Input: part model. Units: mm. Frame: model coordinates. A direction names the side the tool comes from. Give positions to 0.01 mm unless a question says otherwise; leave off trailing zeros. Loops run counter-clockwise (first coordinate to the right, second up) from the corner with the lowest first, then second, coordinate; pieces in that order, holes last. Notation, with made-up numbers: (65, 49) - (84, 49) arc R22 ccw to (84, 76) - close; hole circle Ø10 at (82.25, 60). An arc over 180 degrees is marked (long way). Answer as a JSON object with one key per item and string values.
from build123d import *

# Parameters (mm, degrees)
F1_DEPTH = 288
F3_DEPTH = 304
F5_W     = 50.8
F5_H     = 304
F6_DEPTH = 36
F7_W     = 75.9582033121
F7_H     = 107.4988492727
F8_DEPTH = 100
F9_R     = 10


with BuildPart() as f1:
    # F0 (on Front) → F1 (new body)
    with BuildSketch(Plane.XZ):
        Polygon((0, 48.8444454968), (0, 0), (134.5802352905, 0), (134.5802352905, 40), (62.8, 64.8444454968), (50.8, 64.8444454968), (50.8, 48.8444454968), align=None)
    extrude(amount=F1_DEPTH)

    # F2 (on Front) → F3 (join)
    with BuildSketch(Plane.XZ):
        Polygon((0, 0), (134.5802352905, 0), (134.5802352905, 40), (62.8, 64.8444454968), (0, 64.8444454968), align=None)
    extrude(amount=-F3_DEPTH)

    # F5 (on face) → F6 (join)
    with BuildSketch(Plane.XY.offset(64.8444454968)):
        with Locations((25.4, 152)):
            Rectangle(F5_W, F5_H)
    extrude(amount=F6_DEPTH)

    # F7 (on face) → F8 (join)
    with BuildSketch(Plane(origin=(26.7612103496, 0, 77.3181263313), x_dir=(0.944996487, 0, -0.3270804787), z_dir=(0.3270804787, 0, 0.944996487))):
        with Locations((76.1155287701, 250.2505753636)):
            Rectangle(F7_W, F7_H)
    extrude(amount=F8_DEPTH)

    # F9
    f9_edges = [f1.edges().sort_by_distance(p)[0] for p in [
        (62.8, 250.250575, 64.844445),
    ]]
    fillet(f9_edges, radius=F9_R)


solid = f1.part
Item 1: Cut plane C-C (z = 83). Return loops of the section in (x, y).
Geometry check:
{"outline": "(0, 0) - (50.8, 0) - (50.8, 304) - (0, 304) - close; (69.08, 196.5) - (149.46, 196.5) - (149.46, 304) - (69.08, 304) - close"}
Item 2: Access query for faces 5 (the face through (119, 196.501, 96)), 6 (the face through (25, 154, 100.844)), 7 (the face through (50.8, -142, 57)), 8 (the face through (134.58, 4, 20)). Directions: +Z, -Z, +X, -X, +Y, -Y. A direction counts if a zero-diameter tool reaches every point of the face in a straight line with its end or side. Return the directions, or none.
Geometry check:
{"face 5": "+Z, +X, -Y", "face 6": "+Z, -X, +Y, -Y", "face 7": "+Z, -X, -Y", "face 8": "-Z, +X, +Y, -Y"}
Item 3: Cut plane B-B (x = 11). Return loops of the section in (y, z).
Geometry check:
{"outline": "(-288, 0) - (304, 0) - (304, 100.84) - (0, 100.84) - (0, 48.84) - (-288, 48.84) - close"}
Item 4: Cut plane A-A (y = -249). Return loops of the section in (x, z), then the cut area to 3 significant figures.
Geometry check:
{"outline": "(0, 0) - (134.58, 0) - (134.58, 40) - (62.8, 64.84) - (50.8, 64.84) - (50.8, 48.84) - (0, 48.84) - close", "area": "7,020 mm2"}
Item 5: Cut plane D-D (z = 30.5). Return loops of the section in (x, y), then the cut area to 3 significant figures.
Geometry check:
{"outline": "(0, -288) - (134.58, -288) - (134.58, 304) - (0, 304) - close", "area": "79,700 mm2"}
Item 6: Contact query for flat-ended pins moving along their axis: P1, Ø8, axis at x = 69, y = 29, coming from the +Z side; P2, Ø9.5, axis at x = 55.5, y = -29.5, coming from the +Z side; P3, Ø6, axis at x = 89.5, y = -53, coming from the +Z side. Output: stop coordinate, or through.
Geometry check:
{"P1": "stops at z = 64.08", "P2": "stops at z = 64.84", "P3": "stops at z = 56.64"}
Item 7: Material intervals for line 1 (Z direction, x = 31, y = -235); line 2 (X direction, y = -194, z = 21); line 3 (Y direction, x = 75, z = 98.5), sorted ascending. Write a range as [from, to].
Geometry check:
{"line 1": "z = [0, 48.84]", "line 2": "x = [0, 134.58]", "line 3": "y = [196.5, 304]"}
Item 8: Mould query, pull axis X, two halves, no side actions, for faces 1 (the face through (50.8, 150, 83)), 2 (the face through (0, 70, 39)), 3 (the face through (80.106, 249.498, 114.844)), 4 (the face through (66, -288, 26)). Classes: released by +X, released by -X, zero draft, split by the parting line, or undercut.
Geometry check:
{"face 1": "undercut", "face 2": "released by -X", "face 3": "undercut", "face 4": "zero draft"}
